Work out the finished part from the listing and answer in its coordinate system (mm). A direction names the side the tool comes from. Coordinates: 2 decimals unless noted, no trailing zeros. Order: outer loops, then holes, each group sorted by start corner. A loop starts at its lowest first (then second) coordinate and runs counter-clockwise, first axis right, second up. Notation, with made-up numbers: (1.25, -3.5) -> (58.25, -3.5) arc R16 ccw to (58.25, 7.5) -> close; hole circle Ø10 at (45, 54). An arc over 180 degrees is marked (long way). Use one line per item in the form item = value.
from build123d import *

# Parameters (mm, degrees)
SKETCH2_R          = 6.35
LENGTH_DEPTH       = 31.75
CUT_EXTRUDE1_DEPTH = 4.3688


with BuildPart() as part:
    # Sketch1 → Head (revolve)
    with BuildSketch(Plane.XY):
        Polygon((0, 6.3754), (11.509375, 6.3754), (11.509375, 5.935182001), (6.35, 0), (0, 0), align=None)
    revolve(axis=Axis((0, -1.82358767, 0), (0, 1, 0)))

    # Sketch2 → Length (add)
    with BuildSketch(Plane(origin=(0, 0, 0), x_dir=(1, 0, 0), z_dir=(0, 1, 0))):
        Circle(SKETCH2_R)
    extrude(amount=-LENGTH_DEPTH)

    # Sketch3 → Cut-Extrude1 (cut)
    with BuildSketch(Plane(origin=(0, 6.3754, 0), x_dir=(-1, 0, 0), z_dir=(0, 1, 0))):
        Polygon((2.291358881, 3.96875), (-2.291358881, 3.96875), (-4.582717762, 0), (-2.291358881, -3.96875), (2.291358881, -3.96875), (4.582717762, 0), align=None)
    extrude(amount=-CUT_EXTRUDE1_DEPTH, mode=Mode.SUBTRACT)


solid = part.part
(1) Section B-B on y = -21 is taken. Write down the section's boundary in (x, z), plus the area to 3 significant figures.
Data:
outline = circle Ø12.7 at (0, 0)
area = 127 mm²
(2) Which of the six approach directions +Z, -Z, +X, -X, +Y, -Y give full straight-line access (tool end or side, diameter ignored) to faces 4 (the flat face through (3.45, 4.22, -1.96)), 5 (the flat face through (0, -31.75, 0)), 6 (the cylindrical face through (-1.38, -15.65, 6.2))?
Data:
face_4 = +Y
face_5 = +Z, -Z, +X, -X, -Y
face_6 = -Y
(3) Section A-A on x = 0 is taken. Write down the section's boundary in (y, z).
Data:
outline = (-31.75, -6.35) -> (0, -6.35) -> (5.94, -11.51) -> (6.38, -11.51) -> (6.38, -3.97) -> (2.01, -3.97) -> (2.01, 3.97) -> (6.38, 3.97) -> (6.38, 11.51) -> (5.94, 11.51) -> (0, 6.35) -> (-31.75, 6.35) -> close
(4) Section C-C on y = 1.5 is taken. Write down the section's boundary in (x, z).
Data:
outline = circle Ø15.31 at (0, 0)
(5) The mould has two halves that part along Z. Classify faces 1 (the flat face through (3.42, 4.22, 2.01)), 2 (the flat face through (-5, 6.375, 0)), 3 (the cylindrical face through (-9.133, 6.152, 7.003)): released by +Z, released by -Z, zero draft, split by the parting line, or undercut.
Data:
face_1 = undercut
face_2 = zero draft
face_3 = split by the parting line
(6) Straight lines are drawn through the part: line 1 along Y through (x, z) = (-0.5, 0.5); line 2 along Z through (x, y) = (0.25, -19); line 3 along Z through (x, y) = (5.25, -2.5). For each, find the intervals that lie inside material, in ascending order.
Data:
line_1 = -31.75 to 2.01
line_2 = -6.35 to 6.35
line_3 = -3.57 to 3.57
(7) Each of these flat-tipped pins is pushed along its axis until it touches: P1, Ø5, axis at y = -2.5, z = 5.5, coming from the +X side; P2, Ø1.5, axis at x = -5, y = -26.5, coming from the -Z side; P3, Ø1, axis at y = -14, z = -4, coming from the +X side. Where does it stop, or does it pass through?
Data:
P1 = 5.6
P2 = -4.72
P3 = 5.3
